```python
from build123d import *

# Parameters (mm, degrees)
CROQUIS1_W              = 8
CROQUIS1_H              = 8
CROQUIS1_R              = 2.5
SALIENTE_EXTRUIR4_DEPTH = 170


with BuildPart() as part:
    # Croquis1 → Saliente-Extruir4 (new body)
    with BuildSketch(Plane.XY):
        with BuildLine():
            Line((-3, 8.7), (-3, 10))
            Line((-3, 10), (-9, 10))
            ThreePointArc((-9, 10), (-9.707106781, 9.707106781), (-10, 9))
            Line((-10, 9), (-10, 3))
            Line((-10, 3), (-8.7, 3))
            Line((-8.7, 3), (-8.7, 6))
            Line((-8.7, 6), (-4, 3.25))
            Line((-4, 3.25), (-4, 4))
            Line((-4, 4), (-3.25, 4))
            Line((-3.25, 4), (-6, 8.7))
            Line((-6, 8.7), (-3, 8.7))
        make_face()
        with BuildLine():
            Line((9, 10), (3, 10))
            Line((3, 10), (3, 8.7))
            Line((3, 8.7), (6, 8.7))
            Line((6, 8.7), (3.25, 4))
            Line((3.25, 4), (4, 4))
            Line((4, 4), (4, 3.25))
            Line((4, 3.25), (8.7, 6))
            Line((8.7, 6), (8.7, 3))
            Line((8.7, 3), (10, 3))
            Line((10, 3), (10, 9))
            ThreePointArc((10, 9), (9.707106781, 9.707106781), (9, 10))
        make_face()
        with BuildLine():
            Line((10, -9), (10, -3))
            Line((10, -3), (8.7, -3))
            Line((8.7, -3), (8.7, -6))
            Line((8.7, -6), (4, -3.25))
            Line((4, -3.25), (4, -4))
            Line((4, -4), (3.25, -4))
            Line((3.25, -4), (6.25, -8.7))
            Line((6.25, -8.7), (3, -8.7))
            Line((3, -8.7), (3, -10))
            Line((3, -10), (9, -10))
            ThreePointArc((9, -10), (9.707106781, -9.707106781), (10, -9))
        make_face()
        with BuildLine():
            Line((-8.7, -3), (-10, -3))
            Line((-10, -3), (-10, -9))
            ThreePointArc((-10, -9), (-9.707106781, -9.707106781), (-9, -10))
            Line((-9, -10), (-3, -10))
            Line((-3, -10), (-3, -8.7))
            Line((-3, -8.7), (-5.75, -8.7))
            Line((-5.75, -8.7), (-3.25, -4))
            Line((-3.25, -4), (-4, -4))
            Line((-4, -4), (-4, -3.25))
            Line((-4, -3.25), (-8.7, -6))
            Line((-8.7, -6), (-8.7, -3))
        make_face()
        Rectangle(CROQUIS1_W, CROQUIS1_H)
        Circle(CROQUIS1_R, mode=Mode.SUBTRACT)
    extrude(amount=SALIENTE_EXTRUIR4_DEPTH)


solid = part.part
```
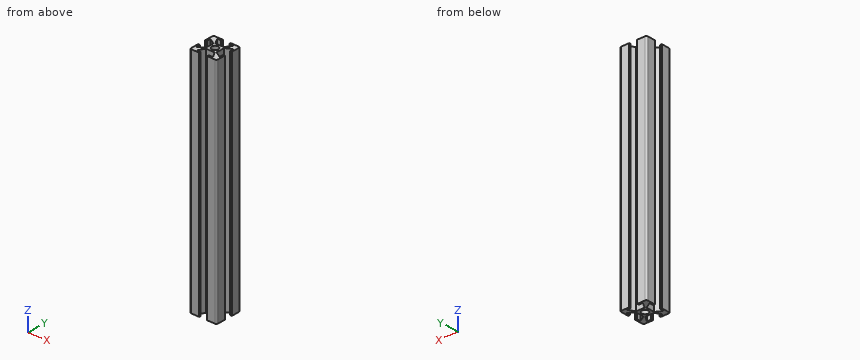
Can you work these out from the model? Positions are in its coordinate system, mm. Coordinates: 2 decimals unless noted, no trailing zeros. Loops run counter-clockwise (first coordinate to the right, second up) from the corner with the lowest first, then second, coordinate; pieces in that order, holes last. Notation, with made-up numbers: (58.5, -8) - (116.5, -8) arc R13 ccw to (116.5, -2) - close; hole circle Ø10 at (-22.75, -38). An arc over 180 degrees is marked (long way). Use a Markdown table: item, result.
Item 1: If I drill on probe 1 along X at (y, z) = (3.25, 153); probe 2 along Y at (x, z) = (0, 102); probe 3 along X at (y, z) = (4.25, 94), over which ranges is the centre line in solid material (lowest first)? Write a range as from..to.
Numbers:
| item | result |
|---|---|
| probe 1 | x = -10..-8.7, -4..4, 8.7..10 |
| probe 2 | y = -4..-2.5, 2.5..4 |
| probe 3 | x = -10..-8.7, -5.71..-3.4, 3.4..5.71, 8.7..10 |
Item 2: I want a section at A-A on x = 0. Please give me the cut outline in (y, z).
Numbers:
| item | result |
|---|---|
| outline | (-4, 0) - (-2.5, 0) - (-2.5, 170) - (-4, 170) - close; (2.5, 0) - (4, 0) - (4, 170) - (2.5, 170) - close |
Item 3: Will these pins go through, and if not, where does the flat tip stop? pin 1 (4 mm diameter, centred on x = 0, y = 0, fed in from -Z); pin 2 (3 mm diameter, centred on x = 0, z = 134, fed in from -Y); pin 3 (0.7 mm diameter, centred on x = -9.5, z = 94.5, fed in from -Y); pin 4 (3 mm diameter, centred on y = -0.5, z = 136.5, fed in from +X).
Numbers:
| item | result |
|---|---|
| pin 1 | passes through |
| pin 2 | stops at y = -4 |
| pin 3 | stops at y = -9.99 |
| pin 4 | stops at x = 4 |
